Work out the finished part from the listing and answer in its coordinate system (mm). A direction names the side the tool comes from. Round coordinates to 2 decimals unless told otherwise and drop trailing zeros. Loops run counter-clockwise (first coordinate to the right, second up) from the corner with the lowest first, then second, coordinate; pieces in that order, holes last.
```python
from build123d import *

# Parameters (mm, degrees)
SKETCH1_W            = 25.4
SKETCH1_H            = 28.575
BOSS_EXTRUDE1_DEPTH  = 3.175
SKETCH2_W            = 25.4
SKETCH2_H            = 3.175
BOSS_EXTRUDE2_DEPTH  = 25.4
SKETCH4_R            = 1.4097
CUT_EXTRUDE1_DEPTH   = 29.575
LPATTERN1_COUNT      = 2
LPATTERN1_PITCH      = 10.16
LPATTERN1_COUNT_DIR2 = 2
LPATTERN1_PITCH_DIR2 = 10.16
SKETCH5_R            = 1.4097
CUT_EXTRUDE2_DEPTH   = 4.175


with BuildPart() as part:
    # Sketch1 → Boss-Extrude1 (new body)
    with BuildSketch(Plane.XY):
        Rectangle(SKETCH1_W, SKETCH1_H)
    extrude(amount=BOSS_EXTRUDE1_DEPTH)

    # Sketch2 → Boss-Extrude2 (add)
    with BuildSketch(Plane.XY.offset(3.175)):
        with Locations((0, -12.7)):
            Rectangle(SKETCH2_W, SKETCH2_H)
    extrude(amount=BOSS_EXTRUDE2_DEPTH)

    # Sketch4 → Cut-Extrude1 (cut, through all)
    with BuildSketch(Plane(origin=(0, 0, 0), x_dir=(-1, 0, 0), z_dir=(0, 0, -1))):
        with Locations((-5.08, 6.0325)):
            Circle(SKETCH4_R)
    cut_extrude1 = extrude(amount=-CUT_EXTRUDE1_DEPTH, mode=Mode.SUBTRACT)

    # LPattern1: Cut-Extrude1 2 × 2
    with Locations(*[(-j * LPATTERN1_PITCH_DIR2, -i * LPATTERN1_PITCH, 0) for i in range(LPATTERN1_COUNT) for j in range(LPATTERN1_COUNT_DIR2) if (i, j) != (0, 0)]):
        add(cut_extrude1, mode=Mode.SUBTRACT)

    # Sketch5 → Cut-Extrude2 (cut, through all)
    with BuildSketch(Plane(origin=(0, -11.1125, 0), x_dir=(1, 0, 0), z_dir=(0, 1, 0))):
        with Locations((-5.08, -20.955)):
            Circle(SKETCH5_R)
    extrude(amount=-CUT_EXTRUDE2_DEPTH, mode=Mode.SUBTRACT)


solid = part.part
```
1. Consider probe 1 along Y at (x, z) = (5.08, 1.6); probe 2 along Y at (x, z) = (-5.5, 2.5); probe 3 along Z at (x, y) = (6.25, -10) (3 decimals). Determine where each line is inside the solid, lowest interval first.
Answer key:
probe 1: y = -14.29 to -5.54, -2.72 to 4.62, 7.44 to 14.29
probe 2: y = -14.29 to -5.47, -2.78 to 4.69, 7.38 to 14.29
probe 3: z = 0 to 3.175
2. Given pin 1 (12.5 mm diameter, centred on x = 0.5, z = 20, fed in from +Y); pin 2 (4.5 mm diameter, centred on x = -5.08, y = -4.13, fed in from -Z); pin 3 (2.5 mm diameter, centred on x = -5.08, z = 20.955, fed in from +Y); pin 4 (7.5 mm diameter, centred on x = -1, y = 6, fed in from +Z) (3 decimals), each flat-ended and moving along its own axis, determine where each tip first touches the part or whether it passes through.
Answer key:
pin 1: stops at y = -11.11
pin 2: stops at z = 0
pin 3: passes through
pin 4: stops at z = 3.175
3. Find section B-B (x = -5.08). Write down the section's boundary in (y, z) (1 decimal), then the cut area to 3 significant figures.
Answer key:
outline: (-14.3, 0) - (-5.5, 0) - (-5.5, 3.2) - (-11.1, 3.2) - (-11.1, 19.5) - (-14.3, 19.5) - close; (-14.3, 22.4) - (-11.1, 22.4) - (-11.1, 28.6) - (-14.3, 28.6) - close; (-2.7, 0) - (4.6, 0) - (4.6, 3.2) - (-2.7, 3.2) - close; (7.4, 0) - (14.3, 0) - (14.3, 3.2) - (7.4, 3.2) - close
area: 145 mm2
4. Find section C-C (y = -3.5). Write down the section's boundary in (x, z) (3 decimals).
Answer key:
outline: (-12.7, 0) - (-6.342, 0) - (-6.342, 3.175) - (-12.7, 3.175) - close; (-3.818, 0) - (3.818, 0) - (3.818, 3.175) - (-3.818, 3.175) - close; (6.342, 0) - (12.7, 0) - (12.7, 3.175) - (6.342, 3.175) - close
5. Determine the mould class of faces 3 (the face through (4.32, 7.22, 1.57)), 4 (the face through (0, 2, 3.175)), 5 (the face through (12.7, -12, 8)) for opening direction X: +X half, -X half, draft (parallel to the pull), parting line (faces both ways), or undercut.
Answer key:
face 3: undercut
face 4: draft
face 5: +X half
6. Find section D-D (z = 20.5). Write down the section's boundary in (x, y).
Answer key:
outline: (-12.7, -14.29) - (-6.41, -14.29) - (-6.41, -11.11) - (-12.7, -11.11) - close; (-3.75, -14.29) - (12.7, -14.29) - (12.7, -11.11) - (-3.75, -11.11) - close
7. Find section A-A (x = 5.08). Write down the section's boundary in (y, z) (1 decimal).
Answer key:
outline: (-14.3, 0) - (-5.5, 0) - (-5.5, 3.2) - (-11.1, 3.2) - (-11.1, 28.6) - (-14.3, 28.6) - close; (-2.7, 0) - (4.6, 0) - (4.6, 3.2) - (-2.7, 3.2) - close; (7.4, 0) - (14.3, 0) - (14.3, 3.2) - (7.4, 3.2) - close
8. Which of the six approach directions +Z, -Z, +X, -X, +Y, -Y give full straight-line access (tool end or side, diameter ignored) to faces 1 (the face through (0, 14.288, 2)), 2 (the face through (0, -11.112, 16))?
Answer key:
face 1: +Z, -Z, +X, -X, +Y
face 2: +Z, +X, -X, +Y
